Autodesk Inventor part; units mm, degrees
ref_plane "YZ Plane" through (0, 0, 0) normal (1, 0, 0) x (0, 1, 0)
ref_plane "XZ Plane" through (0, 0, 0) normal (0, 1, 0) x (-1, 0, 0)
ref_plane "XY Plane" through (0, 0, 0) normal (0, 0, 1) x (1, 0, 0)
sketch "スケッチ1" plane through (0, 0, 0) normal (0, 0, 1) x (1, 0, 0)
  line L0 (0, 0) -> (45, 0)
  line L1 (45, 0) -> (45, 100)
  line L2 (45, 100) -> (0, 100)
  line L3 (0, 100) -> (0, 0)
  dimension "d0" = 100
  dimension "d1" = 45
extrude "押し出し1" add sketch "スケッチ1" along normal blind 7
sketch "スケッチ2" plane through (0, 0, 7) normal (0, 0, 1) x (1, 0, 0)
  line L0 (0, 0) -> (45, 0)
  point P0 (22.6447, 79.5)
  dimension "d4" = 79.5
hole "穴1" at (22.6447, 79.5, 7) direction (0, 0, -1) diameter 12.5 end through all
sketch "スケッチ3" plane through (0, 0, 0) normal (0, 0, -1) x (-1, 0, 0)
  line L0 (0, 0) -> (-45, 0)
  line L1 (-45, 0) -> (-45, 100)
  line L2 (0, 100) -> (0, 0)
  point P0 (-10, 10)
  point P1 (-35, 10)
  dimension "d12" = 10
  dimension "d13" = 10
  dimension "d14" = 10
  dimension "d15" = 10
hole "穴2" at (10, 10, 0) at (35, 10, 0) direction (0, 0, 1) diameter 5 end through all
sketch "スケッチ4" plane through (0, 0, 0) normal (0, 0, -1) x (-1, 0, 0)
  point P0 (0, 0)
properties part number "回転軸取り付け板"
Can you work these out from the model? Positions are in its coordinate system, mm. Coordinates: 2 decimals unless noted, no trailing zeros. Order: outer loops, then holes, each group sorted by start corner. A loop starts at its lowest first (then second) coordinate and runs counter-clockwise, first axis right, second up.
1. If we section it at B-B (y = 79.5): Please give me the cut outline in (x, z).
2. If we section it at D-D (z = 4.25): Please give me the cut outline in (x, y).
3. Thinking about a two-plate mould opening in X: for faces 1 (the face through (20.767, 73.539, 3.451)), 2 (the face through (22, 0, 3)), 3 (the face through (32.89, 11.34, 3.55)), 4 (the face through (0, 51, 3)), which applies, +X half, -X half, draft (parallel to the pull), parting line (faces both ways), or undercut?
4. If we section it at A-A (x = 35): Please give me the cut outline in (y, z), then the cut area to 3 significant figures.
5. I need wall thicknesses on line 1 (X direction, y = 10, z = 2.5); line 2 (X direction, y = 79.5, z = 2.5); line 3 (Y direction, x = 10, z = 1.75). Which ranges of each line are inside material? Lowest first, please.
6. I'm going to push a flat-ended pin straight in: pin 1 (7.5 mm diameter, centred on x = 22.64, y = 79.5, fed in from +Z). Where does the tip first touch, or does it pass through?
7. If we section it at C-C (y = 10): Please give me the cut outline in (x, z), then the cut area to 3 significant figures.
Entries:
1. outline: (0, 0) - (16.39, 0) - (16.39, 7) - (0, 7) - close; (28.89, 0) - (45, 0) - (45, 7) - (28.89, 7) - close
2. outline: (0, 0) - (45, 0) - (45, 100) - (0, 100) - close; hole circle Ø5 at (10, 10); hole circle Ø12.5 at (22.64, 79.5); hole circle Ø5 at (35, 10)
3. face 1: undercut
3. face 2: draft
3. face 3: undercut
3. face 4: -X half
4. outline: (0, 0) - (7.5, 0) - (7.5, 7) - (0, 7) - close; (12.5, 0) - (100, 0) - (100, 7) - (12.5, 7) - close
4. area: 665 mm2
5. line 1: x = 0 to 7.5, 12.5 to 32.5, 37.5 to 45
5. line 2: x = 0 to 16.39, 28.89 to 45
5. line 3: y = 0 to 7.5, 12.5 to 100
6. pin 1: passes through
7. outline: (0, 0) - (7.5, 0) - (7.5, 7) - (0, 7) - close; (12.5, 0) - (32.5, 0) - (32.5, 7) - (12.5, 7) - close; (37.5, 0) - (45, 0) - (45, 7) - (37.5, 7) - close
7. area: 245 mm2
